Part print with two shaded views. Sizes in mm from the minimum x, y, z corner. A direction names the side the tool comes from. Round coordinates to 2 decimals unless told otherwise and drop trailing zeros. Use one line per item in the form item = value. Start each with the question number.
Item 1: Tool access for the marked faces 4, 5 and 6: list every direction of +Z, -Z, +X, -X, +Y, -Y with a clear straight run to the whole face (end or side of a thin tool).
Item 2: Pull direction Z, two halves, no side cores. Call the marked faces 1, 2 and 3: +Z half, -Z half, draft (parallel to the pull), parting line (faces both ways), or undercut.
Item 3: Pin check, flat tips, straight feed: pin 1 (5 mm diameter, centred on y = 6, z = 2.5, fed in from -X) (3 decimals); pin 2 (1.5 mm diameter, centred on y = 29, z = 2, fed in from +X); pin 3 (4 mm diameter, centred on y = 9, z = 3.5, fed in from +X) (3 decimals); pin 4 (5 mm diameter, centred on x = 4, z = 4, fed in from -Y). Stop position of each tip, or through.
Item 4: Drill centre lines: L1, parallel to Y at x = 8, z = 3; L2, parallel to Z at x = 8, y = 35.5; L3, parallel to Y at x = 5.25, z = 6. Where is each one in solid material? Low to high.
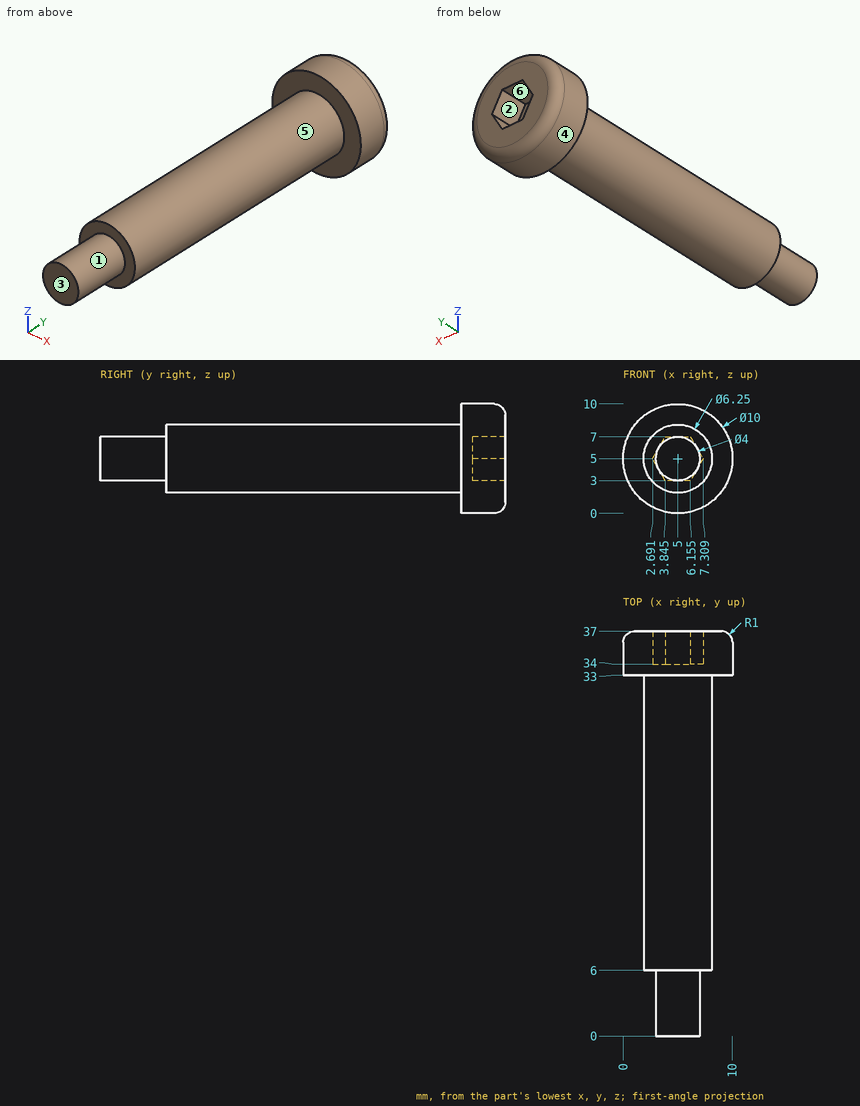
Determined:
q1.face_4 = +Y, -Y
q1.face_5 = -Y
q1.face_6 = +Y
q2.face_1 = parting line
q2.face_2 = undercut
q2.face_3 = draft
q3.pin_1 = 1.875
q3.pin_2 = 7.17
q3.pin_3 = 8.125
q3.pin_4 = 0
q4.L1 = 33 to 37
q4.L2 = 1 to 9
q4.L3 = 0 to 34
